```python
from build123d import *

# Parameters (mm, degrees)
BOSS_EXTRU_2_DEPTH      = 3
ENL_V_MAT_EXTRU_1_DEPTH = 141.768934672
EMPREINTE1_START        = 63.105178129
EMPREINTE1_DEPTH        = 3
EMPREINTE1_START_2      = 93.105178129
EMPREINTE1_2_DEPTH      = 3


# Read off the part's stored shape, not the designer's step: Empreinte1
with BuildPart() as part:
    # Esquisse1 → Boss.-Extru.2 (new body)
    with BuildSketch(Plane.XY):
        with BuildLine():
            Line((40.247233076, 111.105178129), (40.247233076, 61.105178129))
            ThreePointArc((40.247233076, 61.105178129), (44.191308202, 49.180108885), (54.467960723, 41.95837654))
            add(Edge.make_bspline(
                [(54.467960723, 41.95837654), (93.469157599, 30.186251687), (94.060386504, -42.130931626), (70.625681641, -69.023414216)],
                knots=[0.073601613, 0.073601613, 0.073601613, 0.073601613, 1, 1, 1, 1], degree=3))
            Line((70.625681641, -69.023414216), (63.086562616, -62.453658944))
            add(Edge.make_bspline(
                [(51.578324546, 32.384975746), (52.441823747, 32.124337068), (54.160244695, 31.504173294), (57.306848095, 29.97035453), (60.909260152, 27.464002891), (64.778911343, 23.487842732), (69.333722485, 16.888912111), (73.713189985, 6.383804922), (76.439302823, -8.617528818), (76.523407917, -21.892716717), (75.336804817, -32.248132674), (73.851279993, -39.698340102), (71.811754469, -46.646923176), (69.699842941, -51.863805262), (67.806756273, -55.601272185), (66.298875889, -58.166006571), (64.985680603, -60.08494816), (63.904092742, -61.488799964), (63.366023798, -62.13296342), (63.086562616, -62.453658944)],
                knots=[0.073601613, 0.073601613, 0.073601613, 0.073601613, 0.102551563, 0.131501512, 0.189401411, 0.247301311, 0.30520121, 0.421001008, 0.536800806, 0.652600605, 0.710500504, 0.768400403, 0.826300302, 0.884200202, 0.913150151, 0.942100101, 0.97105005, 0.985525025, 1, 1, 1, 1], degree=3))
            ThreePointArc((51.578324546, 32.384975746), (36.163345766, 43.217574263), (30.247233076, 61.105178129))
            Line((30.247233076, 61.105178129), (30.247233076, 111.105178129))
            Line((30.247233076, 111.105178129), (40.247233076, 111.105178129))
        make_face()
    extrude(amount=BOSS_EXTRU_2_DEPTH)

    # Esquisse2 → Enlèv. mat.-Extru.1 (cut, through all)
    with BuildSketch(Plane.XY.offset(3)):
        with BuildLine():
            Line((58.604840791, -65.718091867), (72.675095618, -21.396789164))
            Line((72.675095618, -21.396789164), (77.883188433, -27.569343611))
            ThreePointArc((77.883188433, -27.569343611), (79.106345528, -28.256142913), (80.479757382, -27.970579539))
            Line((80.479757382, -27.970579539), (87.91787168, -23.272823141))
            Line((87.91787168, -23.272823141), (76.157367596, -75.355055511))
            Line((76.157367596, -75.355055511), (58.604840791, -65.718091867))
        make_face()
    extrude(amount=-ENL_V_MAT_EXTRU_1_DEPTH, mode=Mode.SUBTRACT)

    # Empreinte1 outline → Empreinte1 (cut)
    with BuildSketch(Plane(origin=(0, 0, 0), x_dir=(1, 0, 0), z_dir=(0, 1, 0)).offset(EMPREINTE1_START)):
        with BuildLine():
            ThreePointArc((40.222725568, -0.2), (40.219098005, -0.099995306), (40.215220265, 0))
            Line((40.215220265, 0), (30.247233076, 0))
            Line((30.247233076, 0), (30.247233076, -3))
            Line((30.247233076, -3), (35.247233076, -3))
            Line((35.247233076, -3), (35.247233076, -0.2))
            Line((35.247233076, -0.2), (40.222725568, -0.2))
        make_face()
    extrude(amount=EMPREINTE1_DEPTH, mode=Mode.SUBTRACT)

    # Empreinte1 2 outline → Empreinte1 2 (cut)
    with BuildSketch(Plane(origin=(0, 0, 0), x_dir=(1, 0, 0), z_dir=(0, 1, 0)).offset(EMPREINTE1_START_2)):
        with BuildLine():
            ThreePointArc((40.222725568, -0.2), (40.219098005, -0.099995306), (40.215220265, 0))
            Line((40.215220265, 0), (30.247233076, 0))
            Line((30.247233076, 0), (30.247233076, -3))
            Line((30.247233076, -3), (35.247233076, -3))
            Line((35.247233076, -3), (35.247233076, -0.2))
            Line((35.247233076, -0.2), (40.222725568, -0.2))
        make_face()
    extrude(amount=EMPREINTE1_2_DEPTH, mode=Mode.SUBTRACT)


solid = part.part
```
Geometry check sheet. Reference: the model listing, model coordinates, mm. A direction names the side the tool comes from. Coordinates: 2 decimals unless noted, no trailing zeros. Order: outer loops, then holes, each group sorted by start corner. A loop starts at its lowest first (then second) coordinate and runs counter-clockwise, first axis right, second up.
Item 1: Scan lines: line 1 along X through (y, z) = (95, 1.15); line 2 along X through (y, z) = (105.5, 1.55); line 3 along Y through (x, z) = (58.5, 2.95). Record each from-to range of solid material in increasing order.
Item 2: Section check A-A (x = 38). Enter the section's corners in (y, z).
Item 3: Mould release check, pull along Y, two halves, no side actions. Record for faces 1 (the cylindrical face through (44.09, 49.32, 1.48)), 2 (the flat face through (33, 96.105, 1)), 3 (the flat face through (35.247, 65, 2)), 4 (the flat face through (83.28, -26.2, 1.52)): released by +Y, released by -Y, zero draft, split by the parting line, or undercut.
Item 4: Tool access check on faces 5 (the flat face through (35.247, 95, 2)), 6 (the flat face through (38, 65, 0.2)), 7 (the flat face through (40.247, 86, 1)). Record the directions out of +Z, -Z, +X, -X, +Y, -Y that give a thin tool (end or side, any length) a straight path to the whole face; none if there is none.
Item 5: Section check C-C (x = 47.5). Enter the section's corners in (y, z).
Item 6: Section check B-B (y = 52.5). Enter the section's corners in (x, z).
Item 7: Depth check by flat-ended pin: pin 1 (0.9 mm diameter, centred on x = 34, z = 1, fed in from -Y); pin 2 (3.5 mm diameter, centred on x = 39, y = 95.5, fed in from -Z); pin 3 (0.8 mm diameter, centred on y = 64, z = 2, fed in from -X). Enter the tip coordinate at first touch or a pass-through.
Check sheet entries:
1. line 1: x = 35.25 to 40.25
1. line 2: x = 30.25 to 40.25
1. line 3: y = 29.08 to 40.47
2. outline: (40.98, 0) - (63.11, 0) - (63.11, 0.2) - (66.11, 0.2) - (66.11, 0) - (93.11, 0) - (93.11, 0.2) - (96.11, 0.2) - (96.11, 0) - (111.11, 0) - (111.11, 3) - (40.98, 3) - close
3. face 1: released by +Y
3. face 2: undercut
3. face 3: undercut
3. face 4: released by -Y
4. face 5: +Z, -Z, -X
4. face 6: -Z, -X
4. face 7: +Z, -Z, +X, +Y
5. outline: (33.95, 0) - (45.69, 0) - (45.69, 3) - (33.95, 3) - close
6. outline: (31.51, 0) - (42.19, 0) - (42.19, 3) - (31.51, 3) - close
7. pin 1: stops at y = 45.79
7. pin 2: stops at z = 0
7. pin 3: stops at x = 35.25
